Study the drawing (mm; zero at the part's minimum x, y, z) and answer. Coordinates: 2 decimals unless noted, no trailing zeros. Loops run counter-clockwise (first coordinate to the right, second up) from the corner with the lowest first, then second, coordinate; pieces in that order, holes last. Notation, with made-up numbers: (72.5, 81) -> (124.5, 81) arc R24 ccw to (124.5, 108) -> close; hole circle Ø9 at (-32, 1). An arc over 180 degrees is marked (long way). Answer in a Markdown table with one row per item.
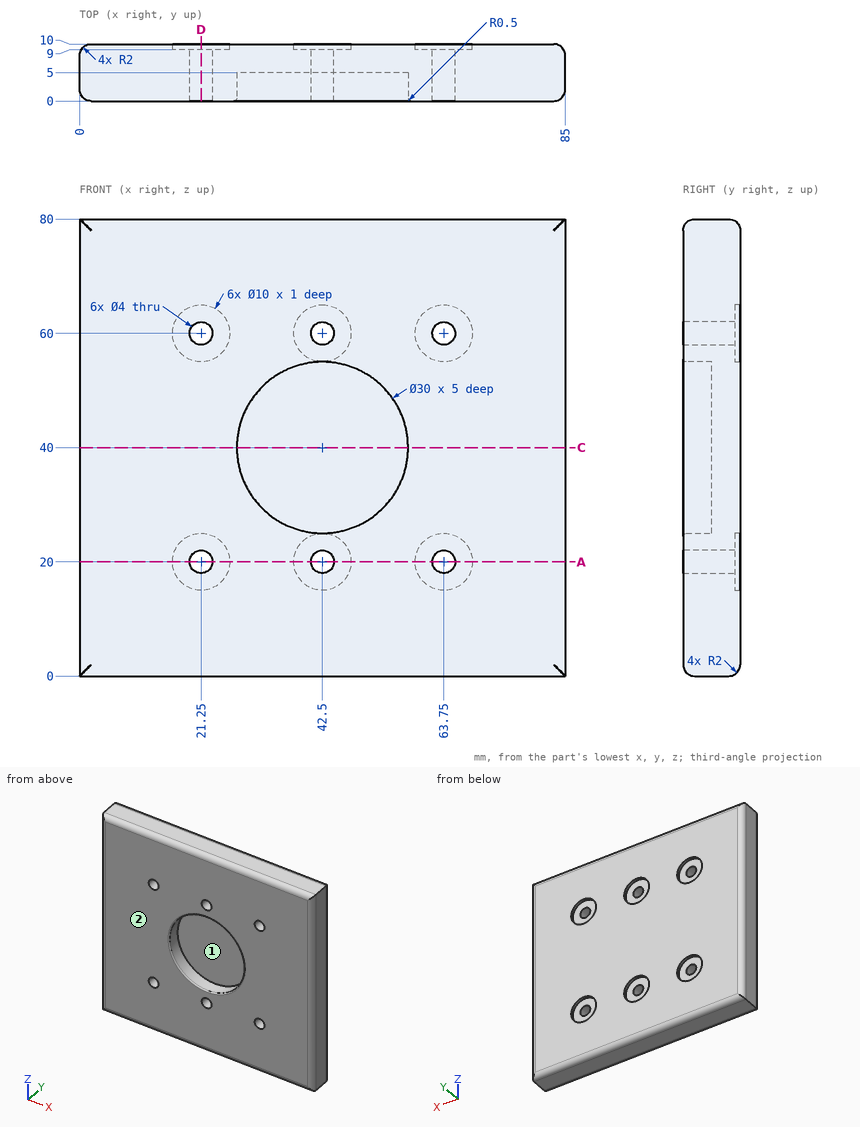
1. The mould has two halves that part along Z. Classify the marked faces 1 and 2: pulls with the +Z half, pulls with the -Z half, needs draft (parallel to the pull), parting line crosses it, or undercut.
A:
| item | result |
|---|---|
| face 1 | undercut |
| face 2 | needs draft |
2. Given pin 1 Ø9 at (x, z) = (48, 39.5) entering from -Y; pin 2 Ø6 at (x, z) = (42.5, 60) entering from +Y, each flat-ended and moving along its own axis, determine where each tip first touches the part or whether it passes through.
A:
| item | result |
|---|---|
| pin 1 | stops at y = 5 |
| pin 2 | stops at y = 9 |
3. Find the intervals of material crossed by probe 1 along X at (y, z) = (3.75, 20); probe 2 along X at (y, z) = (9.8, 60); probe 3 along X at (y, z) = (1.85, 40), in increasing order.
A:
| item | result |
|---|---|
| probe 1 | x = 0 to 19.25, 23.25 to 40.5, 44.5 to 61.75, 65.75 to 85 |
| probe 2 | x = 1.13 to 16.25, 26.25 to 37.5, 47.5 to 58.75, 68.75 to 83.87 |
| probe 3 | x = 0.01 to 27.5, 57.5 to 84.99 |
4. A cutting plane is placed at D-D on x = 21.25. Give the vertices of the cut face in (y, z).
A:
| item | result |
|---|---|
| outline | (0, 2) arc R2 ccw to (2, 0) -> (8, 0) arc R2 ccw to (10, 2) -> (10, 15) -> (9, 15) -> (9, 18) -> (0, 18) -> close; (0, 22) -> (9, 22) -> (9, 25) -> (10, 25) -> (10, 55) -> (9, 55) -> (9, 58) -> (0, 58) -> close; (0, 62) -> (9, 62) -> (9, 65) -> (10, 65) -> (10, 78) arc R2 ccw to (8, 80) -> (2, 80) arc R2 ccw to (0, 78) -> close |
5. A cutting plane is placed at A-A on z = 20. Count the separate pieces of the cut face and the enclosed holes in it, and give its area (3 significant figures).
A:
| item | result |
|---|---|
| separate pieces | 4 |
| enclosed holes | 0 |
| area | 709 mm2 |
6. A cutting plane is placed at C-C on z = 40. Give the vertices of the cut face in (x, y).
A:
| item | result |
|---|---|
| outline | (0, 2) arc R2 ccw to (2, 0) -> (27, 0) arc R0.5 ccw to (27.5, 0.5) -> (27.5, 5) -> (57.5, 5) -> (57.5, 0.5) arc R0.5 ccw to (58, 0) -> (83, 0) arc R2 ccw to (85, 2) -> (85, 8) arc R2 ccw to (83, 10) -> (2, 10) arc R2 ccw to (0, 8) -> close |
